Check sheet for the modelled part. Datum: model origin and axes. Units: mm. Face numbers are marked on the shaded views. A direction names the side the tool comes from. Round coordinates to 2 decimals unless told otherwise and drop trailing zeros. Write each loop counter-clockwise with the first axis right and the second up, starting at its lowest first coordinate (ties: lowest second). Pieces come first, ordered by that corner, then holes.
from build123d import *

# Parameters (mm, degrees)
SKETCH1_W                = 45.4
SKETCH1_H                = 45.4
BOSS_EXTRUDE1_DEPTH      = 12
SKETCH2_W                = 45.4
SKETCH2_H                = 27
CUT_EXTRUDE1_DEPTH       = 10
CUT_EXTRUDE4_REACH       = 67.317
SKETCH13_R               = 1.7
SKETCH20_W               = 7
SKETCH20_H               = 1.4
CUT_EXTRUDE10_DEPTH      = 15
SKETCH21_W               = 10
SKETCH21_H               = 4.8
CUT_EXTRUDE11_DEPTH      = 66.317072806
SKETCH22_W               = 7
SKETCH22_H               = 1.4
CUT_EXTRUDE12_DEPTH      = 15
SKETCH29_W               = 45.4
SKETCH29_H               = 30
BOSS_EXTRUDE6_DEPTH      = 43.5
SKETCH26_W               = 45.4
SKETCH26_H               = 4.4
BOSS_EXTRUDE4_DEPTH      = 16
CUT_EXTRUDE13_DEPTH      = 15
CUT_EXTRUDE13_DEPTH_BACK = 15
SKETCH23_W               = 2
SKETCH23_H               = 7
SKETCH17_R               = 4
CUT_EXTRUDE8_DEPTH       = 78.553658843
CHAMFER1_SIZE2           = 8.242432258
CHAMFER1_SIZE            = 3
CHAMFER2_SIZE2           = 3
CHAMFER2_SIZE            = 8.242432258
SKETCH24_W               = 2
SKETCH24_H               = 9.2
BOSS_EXTRUDE2_DEPTH      = 10.25
SKETCH25_W               = 1.5
SKETCH25_H               = 9.2
BOSS_EXTRUDE3_DEPTH      = 10
FILLET1_R                = 4
CHAMFER3_SIZE            = 3
CHAMFER4_SIZE            = 4.5
SKETCH27_W               = 26.630251868
SKETCH27_H               = 12.344948638
BOSS_EXTRUDE5_DEPTH      = 11.7
SKETCH36_W               = 37.5
SKETCH36_H               = 25
CUT_EXTRUDE18_DEPTH      = 85.867956261
SKETCH28_R               = 1.5
CUT_EXTRUDE14_DEPTH      = 10
SKETCH31_R               = 8
CUT_EXTRUDE15_DEPTH      = 35
SKETCH32_R               = 11.1
CUT_EXTRUDE16_DEPTH      = 27.5
BOSS_EXTRUDE7_DEPTH      = 0.5
SKETCH34_W               = 48
SKETCH34_H               = 47
BOSS_EXTRUDE8_DEPTH      = 2
SKETCH35_R               = 2
SKETCH35_R_2             = 17.5
CUT_EXTRUDE17_DEPTH      = 10
CHAMFER7_SIZE            = 9
CHAMFER7_SIZE2           = 28.544353221


# Some blends are built 0.0001 mm under size
with BuildPart() as part:
    # Sketch1 → Boss-Extrude1 (new body)
    with BuildSketch(Plane.XY):
        with Locations((22.7, 22.7)):
            Rectangle(SKETCH1_W, SKETCH1_H)
    extrude(amount=BOSS_EXTRUDE1_DEPTH)

    # Sketch2 → Cut-Extrude1 (cut)
    with BuildSketch(Plane(origin=(0, 0, 0), x_dir=(-1, 0, 0), z_dir=(0, 0, -1))):
        with Locations((-22.7, 22.7)):
            Rectangle(SKETCH2_W, SKETCH2_H)
    extrude(amount=-CUT_EXTRUDE1_DEPTH, mode=Mode.SUBTRACT)

    # Sketch13 → Cut-Extrude4 (cut, up to next)
    with BuildSketch(Plane.XY.offset(12), mode=Mode.PRIVATE) as cut_extrude4_sk1:
        with Locations((32.7, 32.7)):
            Circle(SKETCH13_R)
    cut_extrude4_tool1 = extrude(cut_extrude4_sk1.sketch, amount=-CUT_EXTRUDE4_REACH, mode=Mode.PRIVATE) & part.part
    # Sketch13 → Cut-Extrude4 (cut, up to next)
    with BuildSketch(Plane.XY.offset(12), mode=Mode.PRIVATE) as cut_extrude4_sk2:
        with Locations((12.7, 32.7)):
            Circle(SKETCH13_R)
    cut_extrude4_tool2 = extrude(cut_extrude4_sk2.sketch, amount=-CUT_EXTRUDE4_REACH, mode=Mode.PRIVATE) & part.part
    # Sketch13 → Cut-Extrude4 (cut, up to next)
    with BuildSketch(Plane.XY.offset(12), mode=Mode.PRIVATE) as cut_extrude4_sk3:
        with Locations((32.7, 12.7)):
            Circle(SKETCH13_R)
    cut_extrude4_tool3 = extrude(cut_extrude4_sk3.sketch, amount=-CUT_EXTRUDE4_REACH, mode=Mode.PRIVATE) & part.part
    # Sketch13 → Cut-Extrude4 (cut, up to next)
    with BuildSketch(Plane.XY.offset(12), mode=Mode.PRIVATE) as cut_extrude4_sk4:
        with Locations((12.7, 12.7)):
            Circle(SKETCH13_R)
    cut_extrude4_tool4 = extrude(cut_extrude4_sk4.sketch, amount=-CUT_EXTRUDE4_REACH, mode=Mode.PRIVATE) & part.part
    add(cut_extrude4_tool1.solids().sort_by_distance((32.7, 32.7, 12))[0], mode=Mode.SUBTRACT)
    add(cut_extrude4_tool2.solids().sort_by_distance((12.7, 32.7, 12))[0], mode=Mode.SUBTRACT)
    add(cut_extrude4_tool3.solids().sort_by_distance((32.7, 12.7, 12))[0], mode=Mode.SUBTRACT)
    add(cut_extrude4_tool4.solids().sort_by_distance((12.7, 12.7, 12))[0], mode=Mode.SUBTRACT)

    # Sketch20 → Cut-Extrude10 (cut)
    with BuildSketch(Plane(origin=(45.4, 0, 0), x_dir=(0, 0, -1), z_dir=(1, 0, 0))):
        with Locations((-3.7, 36.9)):
            Rectangle(SKETCH20_W, SKETCH20_H)
    extrude(amount=-CUT_EXTRUDE10_DEPTH, mode=Mode.SUBTRACT)

    # Sketch21 → Cut-Extrude11 (cut, through all)
    with BuildSketch(Plane(origin=(45.4, 0, 0), x_dir=(0, 0, -1), z_dir=(1, 0, 0))):
        with Locations((-5, 43)):
            Rectangle(SKETCH21_W, SKETCH21_H)
    extrude(amount=-CUT_EXTRUDE11_DEPTH, mode=Mode.SUBTRACT)

    # Sketch22 → Cut-Extrude12 (cut)
    with BuildSketch(Plane.ZY):
        with Locations((3.7, 36.9)):
            Rectangle(SKETCH22_W, SKETCH22_H)
    extrude(amount=-CUT_EXTRUDE12_DEPTH, mode=Mode.SUBTRACT)

    # Sketch29 → Boss-Extrude6 (add)
    with BuildSketch(Plane.XY.offset(12)):
        with Locations((22.7, 15)):
            Rectangle(SKETCH29_W, SKETCH29_H)
    extrude(amount=BOSS_EXTRUDE6_DEPTH)

    # Sketch26 → Boss-Extrude4 (add)
    with BuildSketch(Plane(origin=(0, 0, 0), x_dir=(-1, 0, 0), z_dir=(0, 0, -1))):
        with Locations((-22.7, 38.4)):
            Rectangle(SKETCH26_W, SKETCH26_H)
    extrude(amount=BOSS_EXTRUDE4_DEPTH)

    # Sketch23 → Cut-Extrude13 (cut, two sides: drawn at the far end of the back side and taken through both)
    with BuildSketch(Plane(origin=(0, 40.6, 0), x_dir=(1, 0, 0), z_dir=(0, 1, 0)).offset(-CUT_EXTRUDE13_DEPTH_BACK)):
        with Locations((29.4, -3.7)):
            Rectangle(SKETCH23_W, SKETCH23_H)
        with Locations((16, -3.7)):
            Rectangle(SKETCH23_W, SKETCH23_H)
    extrude(amount=CUT_EXTRUDE13_DEPTH + CUT_EXTRUDE13_DEPTH_BACK, mode=Mode.SUBTRACT)

    # Sketch17 → Cut-Extrude8 (cut, through all)
    with BuildSketch(Plane.XY.offset(12)):
        with Locations((12.7, 32.7)):
            Circle(SKETCH17_R)
        with Locations((32.7, 32.7)):
            Circle(SKETCH17_R)
        with Locations((32.7, 12.7)):
            Circle(SKETCH17_R)
        with Locations((12.7, 12.7)):
            Circle(SKETCH17_R)
    extrude(amount=CUT_EXTRUDE8_DEPTH, mode=Mode.SUBTRACT)

    # Chamfer1
    chamfer1_edges = [part.edges().sort_by_distance(p)[0] for p in [
        (45.4, 40.6, -3),
    ]]
    chamfer1_side = [part.faces().sort_by_distance(p)[0] for p in [
        (45.4, 40.54, -3),
    ]]
    chamfer(chamfer1_edges, length=CHAMFER1_SIZE - 0.0001, length2=CHAMFER1_SIZE2 - 0.0001, reference=chamfer1_side[0])  # a hair under: the kernel refuses the full size

    # Chamfer2
    chamfer2_edges = [part.edges().sort_by_distance(p)[0] for p in [
        (0, 40.6, -3),
    ]]
    chamfer2_side = [part.faces().sort_by_distance(p)[0] for p in [
        (0.06, 40.6, -3),
    ]]
    chamfer(chamfer2_edges, length=CHAMFER2_SIZE - 0.0001, length2=CHAMFER2_SIZE2 - 0.0001, reference=chamfer2_side[0])  # a hair under: the kernel refuses the full size

    # Sketch24 → Boss-Extrude2 (add)
    with BuildSketch(Plane(origin=(0, 0, 0), x_dir=(-1, 0, 0), z_dir=(0, 0, -1))):
        with Locations((-11, 4.6)):
            Rectangle(SKETCH24_W, SKETCH24_H)
    extrude(amount=BOSS_EXTRUDE2_DEPTH)

    # Sketch25 → Boss-Extrude3 (add)
    with BuildSketch(Plane.ZY.offset(-10)):
        with Locations((-9.5, 4.6)):
            Rectangle(SKETCH25_W, SKETCH25_H)
    extrude(amount=BOSS_EXTRUDE3_DEPTH)

    # Fillet1
    fillet1_edges = [part.edges().sort_by_distance(p)[0] for p in [
        (12, 4.6, -10.25),
        (10, 4.6, -8.75),
    ]]
    fillet(fillet1_edges, radius=FILLET1_R)

    # Chamfer3
    chamfer3_edges = [part.edges().sort_by_distance(p)[0] for p in [
        (15, 37.6, 3.7),
        (30.4, 37.6, 3.7),
    ]]
    chamfer(chamfer3_edges, length=CHAMFER3_SIZE - 0.0001)  # a hair under: the kernel refuses the full size

    # Chamfer4
    # the kernel refuses this chamfer: 4.5 mm, written as the material it takes off along each edge
    with BuildSketch(Plane(origin=(28.4, 40.6, 0.2), x_dir=(-0.9996219169112966, 0.027495876610586785, 0), z_dir=(0, 0, 1))) as chamfer4_piece_1:
        Polygon((CHAMFER4_SIZE * 0.999621916911, CHAMFER4_SIZE * 0.0274958766106), (-CHAMFER4_SIZE * 0.0274958766106, CHAMFER4_SIZE * 0.999621916911), (0, 0), align=None)
    extrude(amount=7, mode=Mode.SUBTRACT)
    with BuildSketch(Plane(origin=(17, 40.6, 0.2), x_dir=(0.9996219169112966, 0.027495876610586785, 0), z_dir=(0, 0, 1))) as chamfer4_piece_2:
        Polygon((CHAMFER4_SIZE * 0.999621916911, -CHAMFER4_SIZE * 0.0274958766106), (-CHAMFER4_SIZE * 0.0274958766106, -CHAMFER4_SIZE * 0.999621916911), (0, 0), align=None)
    extrude(amount=7, mode=Mode.SUBTRACT)

    # Sketch27 → Boss-Extrude5 (add)
    with BuildSketch(Plane.XZ.offset(-36.2)):
        with Locations((22.562894264, -9.827525681)):
            Rectangle(SKETCH27_W, SKETCH27_H)
    extrude(amount=BOSS_EXTRUDE5_DEPTH)

    # Sketch36 → Cut-Extrude18 (cut, through all)
    with BuildSketch(Plane(origin=(45.4, 0, 0), x_dir=(0, 0, -1), z_dir=(1, 0, 0))):
        with Locations((-36.75, 15)):
            Rectangle(SKETCH36_W, SKETCH36_H)
    extrude(amount=-CUT_EXTRUDE18_DEPTH, mode=Mode.SUBTRACT)

    # Sketch28 → Cut-Extrude14 (cut)
    with BuildSketch(Plane.XZ.offset(-24.5)):
        with Locations(Location((31.697973452, -9.765616126, 0), (0, 0, 270))):
            Circle(SKETCH28_R)
        with Locations(Location((13.699854881, -9.763930868, 0), (0, 0, 270))):
            Circle(SKETCH28_R)
    extrude(amount=-CUT_EXTRUDE14_DEPTH, mode=Mode.SUBTRACT)

    # Sketch31 → Cut-Extrude15 (cut)
    with BuildSketch(Plane(origin=(0, 30, 0), x_dir=(1, 0, 0), z_dir=(0, 1, 0))):
        with Locations(Location((22.7, -29.5, 0), (0, 0, 270))):
            Circle(SKETCH31_R)
    extrude(amount=-CUT_EXTRUDE15_DEPTH, mode=Mode.SUBTRACT)

    # Sketch32 → Cut-Extrude16 (cut)
    with BuildSketch(Plane.XZ):
        with Locations(Location((22.7, 29.5, 0), (0, 0, 270))):
            Circle(SKETCH32_R)
    extrude(amount=-CUT_EXTRUDE16_DEPTH, mode=Mode.SUBTRACT)

    # Sketch33 → Boss-Extrude7 (add)
    with BuildSketch(Plane.ZY):
        Polygon((10, 45.4), (12, 45.4), (12, 30), (55.5, 30), (55.5, 27.5), (10, 27.5), align=None)
    extrude(amount=BOSS_EXTRUDE7_DEPTH)

    # Sketch34 → Boss-Extrude8 (add)
    with BuildSketch(Plane.ZY.offset(0.5)):
        with Locations((34, 51)):
            Rectangle(SKETCH34_W, SKETCH34_H)
    extrude(amount=BOSS_EXTRUDE8_DEPTH)

    # Sketch35 → Cut-Extrude17 (cut)
    with BuildSketch(Plane.ZY.offset(2.5)):
        with Locations((19.5, 66.5)):
            Circle(SKETCH35_R)
        with Locations((50.5, 66.5)):
            Circle(SKETCH35_R)
        with Locations((50.5, 35.5)):
            Circle(SKETCH35_R)
        with Locations((19.5, 35.5)):
            Circle(SKETCH35_R)
        with Locations((35, 51)):
            Circle(SKETCH35_R_2)
    extrude(amount=-CUT_EXTRUDE17_DEPTH, mode=Mode.SUBTRACT)

    # Chamfer7
    chamfer7_edges = [part.edges().sort_by_distance(p)[0] for p in [
        (-0.5, 45.4, 11),
    ]]
    chamfer7_side = [part.faces().sort_by_distance(p)[0] for p in [
        (22.45, 45.4, 11),
    ]]
    chamfer(chamfer7_edges, length=CHAMFER7_SIZE, length2=CHAMFER7_SIZE2, reference=chamfer7_side[0])


solid = part.part
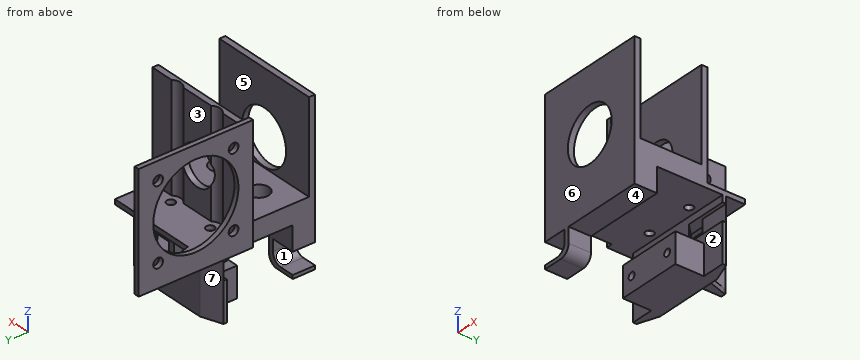
1. Sectioned sample at B-B, the plane x = 26.5. Give the number of separate pieces and of enclosed holes in the cut face, plus the area to 3 significant figures.
2. Sectioned sample at A-A, the plane z = 29.5. Enter the section's corners in (x, y), plus the area to 3 significant figures.
3. Set-up check for the marked faces 1, 2, 3 and 4: record each of +Z, -Z, +X, -X, +Y, -Y from which the full face is reachable in a straight line by a thin tool's end or side.
4. Sectioned sample at D-D, the plane x = 5. Enter the section's corners in (y, z), plus the area to 3 significant figures.
5. Go/stop test with flat-tipped pins: pin 1 (4 mm diameter, centred on y = 6.5, z = -3, fed in from -X); pin 2 (13 mm diameter, centred on x = 23, y = 28.5, fed in from +Z); pin 3 (6.5 mm diameter, centred on x = 2, y = 3.5, fed in from -Z). Record where each tip stops, or that it passes through.
6. Scan lines: line 1 along X through (y, z) = (12.7, 15.8); line 2 along Y through (x, z) = (12.7, 11); line 3 along Y through (x, z) = (16, 50). Record each from-to range of solid material in increasing order.
7. Release check for a two-part mould opening along Y. For the marked faces 5, 6 and 7 record: released by +Y, released by -Y, zero draft, split by the parting line, or undercut.
8. Sectioned sample at C-C, the plane y = 59.5. Enter the section's corners in (x, z).
Computed values:
1. separate pieces: 3
1. enclosed holes: 0
1. area: 704 mm2
2. outline: (-2.5, 27.5) - (14.7, 27.5) - (14.7, 29.24) arc R4 cw to (9.75, 30) - (-0.5, 30) - (-0.5, 34.39) - (-2.5, 34.39) - close; (-2.5, 67.61) - (-0.5, 67.61) - (-0.5, 74.5) - (-2.5, 74.5) - close; (0, 0) - (11.6, 0) - (11.6, 2.5) - (0, 2.5) - close; (30.7, 27.5) - (45.4, 27.5) - (45.4, 30) - (35.65, 30) arc R4 cw to (30.7, 29.24) - close; (33.8, 0) - (45.4, 0) - (45.4, 2.5) - (33.8, 2.5) - close
2. area: 150 mm2
3. face 1: -X, -Y
3. face 2: none
3. face 3: +Z, +X, +Y
3. face 4: -Z, +X, -Y
4. outline: (0, -10.25) - (9.2, -10.25) - (9.2, -8.75) - (0, -8.75) - close; (0, 0) - (9.2, 0) - (9.2, 10) - (36.2, 10) - (36.2, 7.2) - (37.6, 7.2) - (37.6, 0.2) - (36.2, 0.2) - (36.2, -16) - (39.42, -16) - (39.42, 10) - (56.5, 10) - (56.5, 12) - (30, 12) - (30, 55.5) - (27.5, 55.5) - (27.5, 18) - (2.5, 18) - (2.5, 55.5) - (0, 55.5) - close
4. area: 660 mm2
5. pin 1: stops at x = 9.99
5. pin 2: stops at z = 55.5
5. pin 3: stops at z = -10.25
6. line 1: x = 0 to 8.7, 16.7 to 28.7, 36.7 to 45.4
6. line 2: y = 0 to 11, 14.4 to 31, 34.4 to 45.4
6. line 3: y = 0 to 2.5, 27.5 to 30
7. face 5: undercut
7. face 6: released by -Y
7. face 7: released by +Y
8. outline: (-2.5, 10) - (4.05, 10) - (4.05, 12) - (-0.5, 12) - (-0.5, 19.7) - (-2.5, 19.7) - close; (-2.5, 50.3) - (-0.5, 50.3) - (-0.5, 58) - (-2.5, 58) - close
